CAD build for the part. Positions are in the model's coordinates, mm. Face numbers are marked on the shaded views. A direction names the side the tool comes from. Coordinates: 2 decimals unless noted, no trailing zeros. Write each loop counter-clockwise with the first axis right and the second up, starting at its lowest first coordinate (ties: lowest second). Pieces come first, ordered by that corner, then holes. Notation, with made-up numbers: (32.5, -4) - (55.5, -4) arc R17 cw to (55.5, 22) - close; hole circle Ø8 at (82, 23). An arc over 180 degrees is marked (long way). Answer in a Markdown table with one row per item. Add a question column.
Q1. Pin check, flat tips, straight feed: pin 1 (12 mm diameter, centred on x = 66.5, z = 8, fed in from -Y); pin 2 (1.4 mm diameter, centred on y = -1, z = 34.5, fed in from -X); pin 3 (4 mm diameter, centred on y = -3, z = 16.5, fed in from +X). Stop position of each tip, or through.
Q2. Band-saw the part on A-A (z = 5.5). List the corners of the cut face in (x, y), and give its area (3 significant figures).
Q3. Drill centre lines: line 1 along Z through (x, y) = (3.5, -0.75); line 2 along X through (y, z) = (-1.25, 27.5); line 3 along Y through (x, z) = (35.5, 7.5). Where is each one in solid material? Low to high. Write a range as from..to.
Q4. Band-saw the part on C-C (y = -7.5). List the corners of the cut face in (x, z), and give its area (3 significant figures).
Q5. 3-axis set-ups, long thin cutter, end or side, ignore diameter. For the marked faces 1 and 2: which of +Z, -Z, +X, -X, +Y, -Y reach the whole face in a straight line?
Q6. Band-saw the part on B-B (x = 53). List the corners of the cut face in (y, z), and give its area (3 significant figures).
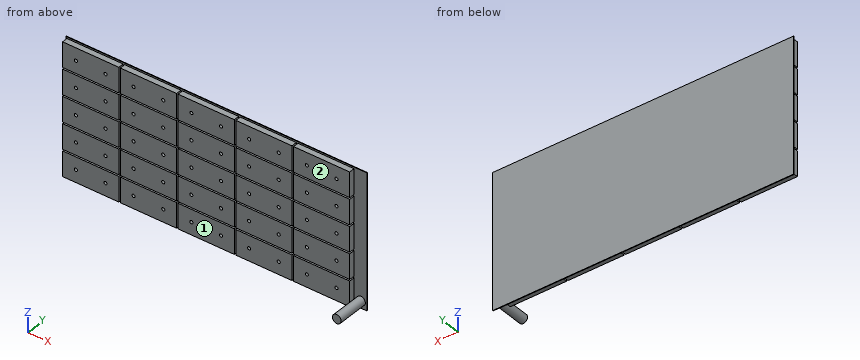
```python
from build123d import *

# Parameters (mm, degrees)
F1_W     = 96.476763
F1_H     = 43.027435
F2_DEPTH = 0.2
F3_R     = 1.408537
F4_DEPTH = 10
F0_W     = 18
F0_H     = 8
F0_R     = 0.5
F5_DEPTH = 2


with BuildPart() as f2:
    # F1 (on Front) → F2 (new body)
    with BuildSketch(Plane.XZ):
        with Locations((38.870699, 16.998278)):
            Rectangle(F1_W, F1_H)
    extrude(amount=F2_DEPTH)

    # F3 (on face) → F4 (join)
    with BuildSketch(Plane.XZ.offset(0.2)):
        with Locations((85.209101, -2.20358)):
            Circle(F3_R)
    extrude(amount=F4_DEPTH)

    # F0 (on Front) → F5 (join)
    with BuildSketch(Plane.XZ):
        Rectangle(F0_W, F0_H)
        with Locations((-4.75, 0)):
            Circle(F0_R, mode=Mode.SUBTRACT)
        with Locations((4.75, 0)):
            Circle(F0_R, mode=Mode.SUBTRACT)
        with Locations((0, 8.5)):
            Rectangle(F0_W, F0_H)
        with Locations((-4.75, 8.5)):
            Circle(F0_R, mode=Mode.SUBTRACT)
        with Locations((4.75, 8.5)):
            Circle(F0_R, mode=Mode.SUBTRACT)
        with Locations((0, 17)):
            Rectangle(F0_W, F0_H)
        with Locations((-4.75, 17)):
            Circle(F0_R, mode=Mode.SUBTRACT)
        with Locations((4.75, 17)):
            Circle(F0_R, mode=Mode.SUBTRACT)
        with Locations((0, 25.5)):
            Rectangle(F0_W, F0_H)
        with Locations((-4.75, 25.5)):
            Circle(F0_R, mode=Mode.SUBTRACT)
        with Locations((4.75, 25.5)):
            Circle(F0_R, mode=Mode.SUBTRACT)
        with Locations((0, 34)):
            Rectangle(F0_W, F0_H)
        with Locations((-4.75, 34)):
            Circle(F0_R, mode=Mode.SUBTRACT)
        with Locations((4.75, 34)):
            Circle(F0_R, mode=Mode.SUBTRACT)
        with Locations((18.5, 0)):
            Rectangle(F0_W, F0_H)
        with Locations((13.75, 0)):
            Circle(F0_R, mode=Mode.SUBTRACT)
        with Locations((23.25, 0)):
            Circle(F0_R, mode=Mode.SUBTRACT)
        with Locations((18.5, 8.5)):
            Rectangle(F0_W, F0_H)
        with Locations((13.75, 8.5)):
            Circle(F0_R, mode=Mode.SUBTRACT)
        with Locations((23.25, 8.5)):
            Circle(F0_R, mode=Mode.SUBTRACT)
        with Locations((18.5, 17)):
            Rectangle(F0_W, F0_H)
        with Locations((13.75, 17)):
            Circle(F0_R, mode=Mode.SUBTRACT)
        with Locations((23.25, 17)):
            Circle(F0_R, mode=Mode.SUBTRACT)
        with Locations((18.5, 25.5)):
            Rectangle(F0_W, F0_H)
        with Locations((13.75, 25.5)):
            Circle(F0_R, mode=Mode.SUBTRACT)
        with Locations((23.25, 25.5)):
            Circle(F0_R, mode=Mode.SUBTRACT)
        with Locations((18.5, 34)):
            Rectangle(F0_W, F0_H)
        with Locations((13.75, 34)):
            Circle(F0_R, mode=Mode.SUBTRACT)
        with Locations((23.25, 34)):
            Circle(F0_R, mode=Mode.SUBTRACT)
        with Locations((37, 0)):
            Rectangle(F0_W, F0_H)
        with Locations((32.25, 0)):
            Circle(F0_R, mode=Mode.SUBTRACT)
        with Locations((41.75, 0)):
            Circle(F0_R, mode=Mode.SUBTRACT)
        with Locations((37, 8.5)):
            Rectangle(F0_W, F0_H)
        with Locations((32.25, 8.5)):
            Circle(F0_R, mode=Mode.SUBTRACT)
        with Locations((41.75, 8.5)):
            Circle(F0_R, mode=Mode.SUBTRACT)
        with Locations((37, 17)):
            Rectangle(F0_W, F0_H)
        with Locations((32.25, 17)):
            Circle(F0_R, mode=Mode.SUBTRACT)
        with Locations((41.75, 17)):
            Circle(F0_R, mode=Mode.SUBTRACT)
        with Locations((37, 25.5)):
            Rectangle(F0_W, F0_H)
        with Locations((32.25, 25.5)):
            Circle(F0_R, mode=Mode.SUBTRACT)
        with Locations((41.75, 25.5)):
            Circle(F0_R, mode=Mode.SUBTRACT)
        with Locations((37, 34)):
            Rectangle(F0_W, F0_H)
        with Locations((32.25, 34)):
            Circle(F0_R, mode=Mode.SUBTRACT)
        with Locations((41.75, 34)):
            Circle(F0_R, mode=Mode.SUBTRACT)
        with Locations((55.5, 0)):
            Rectangle(F0_W, F0_H)
        with Locations((50.75, 0)):
            Circle(F0_R, mode=Mode.SUBTRACT)
        with Locations((60.25, 0)):
            Circle(F0_R, mode=Mode.SUBTRACT)
        with Locations((55.5, 8.5)):
            Rectangle(F0_W, F0_H)
        with Locations((50.75, 8.5)):
            Circle(F0_R, mode=Mode.SUBTRACT)
        with Locations((60.25, 8.5)):
            Circle(F0_R, mode=Mode.SUBTRACT)
        with Locations((55.5, 17)):
            Rectangle(F0_W, F0_H)
        with Locations((50.75, 17)):
            Circle(F0_R, mode=Mode.SUBTRACT)
        with Locations((60.25, 17)):
            Circle(F0_R, mode=Mode.SUBTRACT)
        with Locations((55.5, 25.5)):
            Rectangle(F0_W, F0_H)
        with Locations((50.75, 25.5)):
            Circle(F0_R, mode=Mode.SUBTRACT)
        with Locations((60.25, 25.5)):
            Circle(F0_R, mode=Mode.SUBTRACT)
        with Locations((55.5, 34)):
            Rectangle(F0_W, F0_H)
        with Locations((50.75, 34)):
            Circle(F0_R, mode=Mode.SUBTRACT)
        with Locations((60.25, 34)):
            Circle(F0_R, mode=Mode.SUBTRACT)
        with Locations((74, 0)):
            Rectangle(F0_W, F0_H)
        with Locations((69.25, 0)):
            Circle(F0_R, mode=Mode.SUBTRACT)
        with Locations((78.75, 0)):
            Circle(F0_R, mode=Mode.SUBTRACT)
        with Locations((74, 8.5)):
            Rectangle(F0_W, F0_H)
        with Locations((69.25, 8.5)):
            Circle(F0_R, mode=Mode.SUBTRACT)
        with Locations((78.75, 8.5)):
            Circle(F0_R, mode=Mode.SUBTRACT)
        with Locations((74, 17)):
            Rectangle(F0_W, F0_H)
        with Locations((69.25, 17)):
            Circle(F0_R, mode=Mode.SUBTRACT)
        with Locations((78.75, 17)):
            Circle(F0_R, mode=Mode.SUBTRACT)
        with Locations((74, 25.5)):
            Rectangle(F0_W, F0_H)
        with Locations((69.25, 25.5)):
            Circle(F0_R, mode=Mode.SUBTRACT)
        with Locations((78.75, 25.5)):
            Circle(F0_R, mode=Mode.SUBTRACT)
        with Locations((74, 34)):
            Rectangle(F0_W, F0_H)
        with Locations((69.25, 34)):
            Circle(F0_R, mode=Mode.SUBTRACT)
        with Locations((78.75, 34)):
            Circle(F0_R, mode=Mode.SUBTRACT)
    extrude(amount=F5_DEPTH)


solid = f2.part
```
Checked values:
| question | item | result |
|---|---|---|
| 1 | pin 1 | stops at y = -2 |
| 1 | pin 2 | stops at x = -9 |
| 1 | pin 3 | stops at x = 83 |
| 2 | outline | (-9.37, -0.2) - (-9, -0.2) - (-9, -2) - (9, -2) - (9, -0.2) - (9.5, -0.2) - (9.5, -2) - (27.5, -2) - (27.5, -0.2) - (28, -0.2) - (28, -2) - (46, -2) - (46, -0.2) - (46.5, -0.2) - (46.5, -2) - (64.5, -2) - (64.5, -0.2) - (65, -0.2) - (65, -2) - (83, -2) - (83, -0.2) - (87.11, -0.2) - (87.11, 0) - (-9.37, 0) - close |
| 2 | area | 181 mm² |
| 3 | line 1 | z = -4..4, 4.5..12.5, 13..21, 21.5..29.5, 30..38 |
| 3 | line 2 | x = -9..9, 9.5..27.5, 28..46, 46.5..64.5, 65..83 |
| 3 | line 3 | y = -2..0 |
| 4 | outline | circle Ø2.82 at (85.21, -2.2) |
| 4 | area | 6.23 mm² |
| 5 | face 1 | +Z, -Z, -X, -Y |
| 5 | face 2 | +Z, -Z, +X, -X, -Y |
| 6 | outline | (-2, -4) - (-0.2, -4) - (-0.2, -4.52) - (0, -4.52) - (0, 38.51) - (-0.2, 38.51) - (-0.2, 38) - (-2, 38) - (-2, 30) - (-0.2, 30) - (-0.2, 29.5) - (-2, 29.5) - (-2, 21.5) - (-0.2, 21.5) - (-0.2, 21) - (-2, 21) - (-2, 13) - (-0.2, 13) - (-0.2, 12.5) - (-2, 12.5) - (-2, 4.5) - (-0.2, 4.5) - (-0.2, 4) - (-2, 4) - close |
| 6 | area | 80.6 mm² |
